The listing builds one solid part. Answer for the finished solid, in the listing's coordinates (mm). Face numbers are marked on the shaded views. A direction names the side the tool comes from. Give positions to 0.01 mm unless a question says otherwise; leave off trailing zeros. Loops run counter-clockwise (first coordinate to the right, second up) from the corner with the lowest first, then second, coordinate; pieces in that order, holes last. Notation, with made-up numbers: (-32, 57) - (1, 57) arc R17 cw to (1, 70) - close; hole circle Ø8 at (18, -1). An arc over 180 degrees is marked (long way). Write item = value, one per line. Start each with the question number.
1) The part is cut by section A-A on x = 0. Write down the section's boundary in (y, z), plus the area to 3 significant figures.
2) Consider probe 1 along X at (y, z) = (-1, 8.75); probe 2 along Z at (x, y) = (-2, 17.5); probe 3 along X at (y, z) = (4, 17.75). Determine where each line is inside the solid, lowest interval first.
3) Which of the six approach directions +Z, -Z, +X, -X, +Y, -Y give full straight-line access (tool end or side, diameter ignored) to the marked faces 1 and 2?
4) The part is cut by section C-C on z = 14.5. Write down the section's boundary in (x, y).
5) The part is cut by section D-D on y = 24. Write down the section's boundary in (x, z).
6) Flat-ended cylindrical pins translate along their axes: P1, Ø6, axis at y = 13.5, z = 23.5, coming from the -X side; P2, Ø3, axis at x = -15, y = 3.5, coming from the +Z side; P3, Ø1.5, axis at y = -2.5, z = 5.5, coming from the +X side; P4, Ø1.5, axis at x = -23.5, z = 13, coming from the +Y side. Find the tip coordinate at first contact, or state that the pin passes through.
from build123d import *

# Parameters (mm, degrees)
SKETCH1_R           = 30
BOSS_EXTRUDE3_DEPTH = 12
SKETCH3_R           = 15
BOSS_EXTRUDE4_DEPTH = 17
CHAMFER1_SIZE       = 2


with BuildPart() as part:
    # Sketch1 → Boss-Extrude3 (new body)
    with BuildSketch(Plane.XY):
        Circle(SKETCH1_R)
    extrude(amount=BOSS_EXTRUDE3_DEPTH)

    # Sketch3 → Boss-Extrude4 (add)
    with BuildSketch(Plane.XY.offset(12)):
        Circle(SKETCH3_R)
    extrude(amount=BOSS_EXTRUDE4_DEPTH)

    # Chamfer1
    chamfer1_edges = [part.edges().sort_by_distance(p)[0] for p in [
        (-15, 0, 29),
    ]]
    chamfer(chamfer1_edges, length=CHAMFER1_SIZE)


solid = part.part
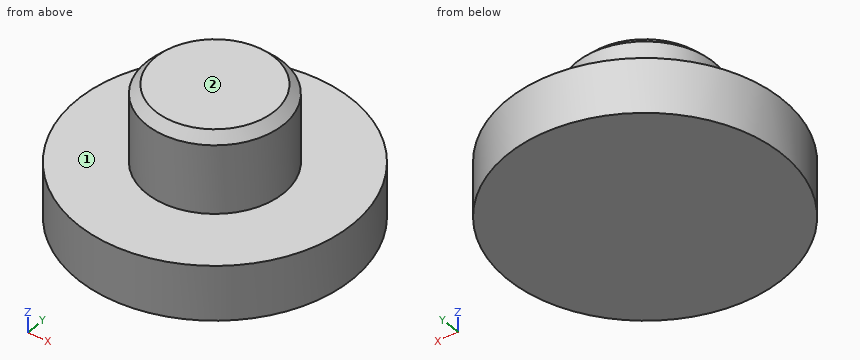
Answer below:
q1.outline = (-30, 0) - (30, 0) - (30, 12) - (15, 12) - (15, 27) - (13, 29) - (-13, 29) - (-15, 27) - (-15, 12) - (-30, 12) - close
q1.area = 1,230 mm2
q2.probe_1 = -29.98 to 29.98
q2.probe_2 = 0 to 12
q2.probe_3 = -14.46 to 14.46
q3.face_1 = +Z
q3.face_2 = +Z, +X, -X, +Y, -Y
q4.outline = circle Ø30 at (0, 0)
q5.outline = (-18, 0) - (18, 0) - (18, 12) - (-18, 12) - close
q6.P1 = -10.71
q6.P2 = 28.1
q6.P3 = 29.95
q6.P4 = through
